Study the drawing (mm; zero at the part's minimum x, y, z) and answer. A direction names the side the tool comes from. Give positions to 0.01 mm unless a question says otherwise; leave off trailing zeros. Write each loop counter-clockwise with the first axis right and the second up, starting at its lowest first coordinate (ties: lowest second). Pieces come first, ordered by that corner, then holes. Notation, with made-up numbers: (-28, 87.25) - (14, 87.25) arc R19 ccw to (14, 104.25) - close; hole circle Ø10 at (24, 76). An arc over 180 degrees is marked (long way). Return JSON: item names as keys, results as strings.
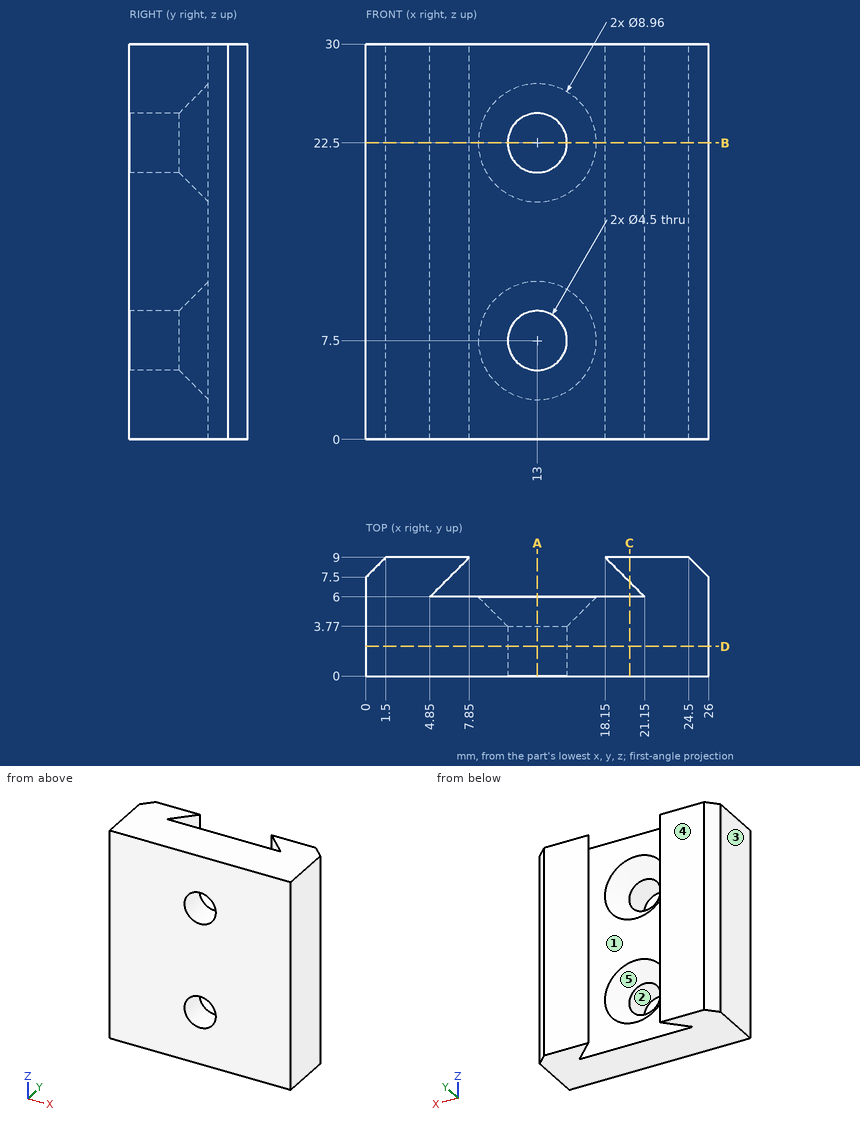
Item 1: A cutting plane is placed at A-A on x = 13. Determine the outline of the cut face in (y, z).
Answer below:
{"outline": "(0, 0) - (6, 0) - (6, 3.02) - (3.77, 5.25) - (0, 5.25) - close; (0, 9.75) - (3.77, 9.75) - (6, 11.98) - (6, 18.02) - (3.77, 20.25) - (0, 20.25) - close; (0, 24.75) - (3.77, 24.75) - (6, 26.98) - (6, 30) - (0, 30) - close"}
Item 2: The mould has two halves that part along X. Classify the marked faces 3, 4 and 5: +X half, -X half, draft (parallel to the pull), parting line (faces both ways), or undercut.
Answer below:
{"face 3": "-X half", "face 4": "draft", "face 5": "undercut"}
Item 3: A cutting plane is placed at D-D on y = 2.25. Determine the outline of the cut face in (x, z).
Answer below:
{"outline": "(0, 0) - (26, 0) - (26, 30) - (0, 30) - close; hole circle Ø4.5 at (13, 7.5); hole circle Ø4.5 at (13, 22.5)"}
Item 4: A cutting plane is placed at C-C on x = 20. Determine the outline of the cut face in (y, z), then the cut area to 4 significant figures.
Answer below:
{"outline": "(0, 0) - (6, 0) - (6, 30) - (0, 30) - close; (7.15, 0) - (9, 0) - (9, 30) - (7.15, 30) - close", "area": "235.5 mm²"}
Item 5: A cutting plane is placed at B-B on z = 22.5. Determine the outline of the cut face in (x, y), then the cut area to 3 significant figures.
Answer below:
{"outline": "(0, 0) - (10.75, 0) - (10.75, 3.77) - (8.52, 6) - (4.85, 6) - (7.85, 9) - (1.5, 9) - (0, 7.5) - close; (15.25, 0) - (26, 0) - (26, 7.5) - (24.5, 9) - (18.15, 9) - (21.15, 6) - (17.48, 6) - (15.25, 3.77) - close", "area": "160 mm²"}
Item 6: Consider L1, parallel to Z at x = 13, y = 1.95; L2, parallel to Z at x = 11.25, y = 5.75; L3, parallel to Y at x = 11.5, z = 17.5. Determine where each line is inside the solid, lowest interval first.
Answer below:
{"L1": "z = 0 to 5.25, 9.75 to 20.25, 24.75 to 30", "L2": "z = 0 to 3.65, 11.35 to 18.65, 26.35 to 30", "L3": "y = 0 to 6"}
Item 7: For the marked faces 1 and 2, determine the directions among +Z, -Z, +X, -X, +Y, -Y from which every point of the face is accessible in a straight line to the end or side of a thin tool.
Answer below:
{"face 1": "+Z, -Z", "face 2": "+Y, -Y"}
